Autodesk Inventor part; units mm, degrees
ref_plane "工作平面1" through (0, 10, 0) normal (0, 1, 0) x (-1, 0, 0)
ref_plane "YZ Plane" through (0, 0, 0) normal (1, 0, 0) x (0, 1, 0)
ref_plane "XY Plane" through (0, 0, 0) normal (0, 0, 1) x (1, 0, 0)
sketch "草图1" plane through (0, 0, 0) normal (0, 1, 0) x (-1, 0, 0)
  line L0 (10, -52.5) -> (-10, -52.5)
  line L1 (-10, -52.5) -> (-10, 52.5)
  line L2 (-10, 52.5) -> (10, 52.5)
  line L3 (10, 52.5) -> (10, -52.5)
  line L4 (10, -52.5) -> (-10, 52.5) construction
  line L5 (-10, -52.5) -> (10, 52.5) construction
  point P0 (0, 0)
  dimension "d0" = 20
  dimension "d1" = 105
extrude "拉伸1" add sketch "草图1" along normal blind 25
sketch "草图3" plane through (0, 25, 0) normal (0, 1, 0) x (1, 0, 0)
  line L0 (10, -52.5) -> (10, 52.5)
  line L1 (10, 52.5) -> (-10, 52.5)
  line L2 (-10, 52.5) -> (-10, -52.5)
  line L3 (-10, 52.5) -> (-10, -52.5)
  line L4 (-10, -52.5) -> (10, -52.5)
  line L5 (10, -52.5) -> (10, 52.5)
  line L6 (-10, 52.5) -> (-10, -28.5)
  line L7 (-10, -24.5) -> (10, -24.5)
  line L8 (10, -52.5) -> (10, 52.5)
  line L9 (10, 52.5) -> (-10, 52.5)
  line L10 (-10, -52.5) -> (10, -52.5)
  point P0 (0, 0)
  point P1 (10, -28.5)
  point P2 (10, -48.5)
  dimension "d12" = 28
extrude "拉伸3" cut sketch "草图3" against normal blind 5 contours L7 L2 L1 L0
sketch "草图4" plane through (0, 20, 0) normal (0, 1, 0) x (1, 0, 0)
  point P0 (0, 0)
sketch "草图6" plane through (0, 0, 0) normal (1, 0, 0) x (0, 1, 0)
  line L0 (0, -52.5) -> (20, -52.5)
  line L1 (0, -52.5) -> (0, 52.5)
  circle A0 centre (10, 4.5) radius 6
  point P0 (0, 0)
  point P1 (15, -52.5)
  dimension "d18" = 57
  dimension "d19" = 10
  dimension "d20" = 12
extrude "拉伸5" cut sketch "草图6" along normal mid plane 19
ref_plane "工作平面1" through (0, 10, 0) normal (0, 1, 0) x (-1, 0, 0)
sketch "草图8" plane through (0, 10, 0) normal (0, 1, 0) x (-1, 0, 0)
  line L0 (10, 52.5) -> (-10, 52.5)
  line L1 (10, -52.5) -> (10, 52.5)
  line L2 (-10, -52.5) -> (10, -52.5)
  line L3 (-10, 52.5) -> (-10, -52.5)
  line L4 (9.5, -1.5) -> (9.5, 10.5)
  line L5 (-9.5, 10.5) -> (-9.5, -1.5)
  line L6 (9.5, -1.5) -> (9.5, 10.5)
  line L7 (9.5, 4.5) -> (10, 4.5)
  line L8 (10, -52.5) -> (10, 52.5)
  line L9 (9.5, -1.5) -> (10, -2)
  line L10 (10, -2) -> (10, 4.5)
  line L11 (9.5, 4.5) -> (9.5, -1.5)
  line L12 (10, 4.5) -> (-10, 4.5)
  line L13 (-10, 52.5) -> (-10, -52.5)
  point P0 (0, 0)
  dimension "d24" = 135
revolve "旋转1" cut sketch "草图8" angle 360 about axis through (-10, 10, 4.5) along (1, 0, 0) contours L1 L9 L4 L7
mirror "镜像1" about plane through (0, 0, 0) normal (1, 0, 0) of "旋转1"
sketch "草图9" plane through (0, 0, 0) normal (1, 0, 0) x (0, 1, 0)
  line L0 (0, -52.5) -> (20, -52.5)
  line L1 (25, 24.5) -> (25, 52.5)
  line L2 (14.5, 38.5) -> (31.5646, 38.5)
  line L3 (14.5, 38.5) -> (14.5, 37)
  line L4 (14.5, 37) -> (16.5, 37)
  line L5 (16.5, 37) -> (25, 28.5)
  line L6 (25, 28.5) -> (25, 38.5)
  line L7 (25, 52.5) -> (25, 24.5)
  line L8 (14.5, 40) -> (16.5, 40)
  line L9 (16.5, 40) -> (25, 48.5)
  line L10 (14.5, 40) -> (14.5, 38.5)
  point P0 (0, 0)
  point P1 (15, -52.5)
  dimension "d26" = 91
  dimension "d27" = 10.5
  dimension "d28" = 1.5
  dimension "d29" = 2
  dimension "d30" = 45
extrude "拉伸6" cut sketch "草图9" along normal through all both and the other way through all
sketch "草图10" plane through (0, 20, 0) normal (0, 1, 0) x (1, 0, 0)
  line L0 (-10, 52.5) -> (-10, -52.5)
  line L1 (-10, 17.5) -> (10, 17.5)
  line L2 (10, -52.5) -> (10, 52.5)
  line L3 (-10, 52.5) -> (10, 52.5)
  circle A0 centre (0, 17.5) radius 7
  line L4 (-7, 17.5) -> (-7, 52.5)
  line L5 (10, 52.5) -> (-10, 52.5)
  line L6 (7, 17.5) -> (6.4266, 52.5)
  point P0 (0, 0)
  point P1 (6.9962, 17.7293)
  dimension "d33" = 35
  dimension "d34" = 14
extrude "拉伸7" cut sketch "草图10" against normal blind 5 contours L3 L6 L1 L4 | L1 A0
properties part number "5-压铁" material "不锈钢"
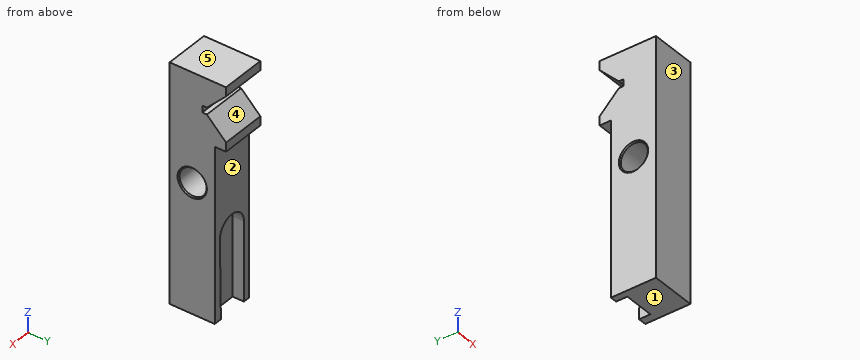
Part model, mm, in its own coordinate system. Face numbers are marked on the shaded views. A direction names the side the tool comes from. Coordinates: 2 decimals unless noted, no trailing zeros. Loops run counter-clockwise (first coordinate to the right, second up) from the corner with the lowest first, then second, coordinate; pieces in that order, holes last. Notation, with made-up numbers: (18.5, -13) - (49.5, -13) arc R13 cw to (49.5, 0) - close; hole circle Ø8 at (80.5, 57.25). An arc over 180 degrees is marked (long way). Write item = value, one per line. Start each with the question number.
Item 1: Cut at A-A, the plane y = 10. Give the cut face in (x, z), and give its area (3 significant figures).
Item 2: Cut at D-D, the plane z = 38.5. Give the cut face in (x, y), and give its area (3 significant figures).
Item 3: 3-axis set-ups, long thin cutter, end or side, ignore diameter. For the marked faces 1 and 2: which of +Z, -Z, +X, -X, +Y, -Y reach the whole face in a straight line?
Item 4: Cut at B-B, the plane z = 4.5. Give the cut face in (x, y).
Item 5: Wall check: L1, parallel to Z at x = -5.5, y = 10; L2, parallel to Y at x = -4.75, z = 4.5; L3, parallel to Y at x = -8.25, z = 2. Give the ranges that are in metal, low to high. Write a range as from..to.
Item 6: Mould opens along Z. For the marked faces 3, 4 and 5 say: released by +Z, released by -Z, zero draft, split by the parting line, or undercut.
Item 7: Cut at C-C, the plane x = 0. Give the cut face in (y, z), and give its area (3 significant figures).
Item 8: Flat gauge pins, fed straight in: pin 1 Ø7 at (x, z) = (-2, -28.5) entering from +Y; pin 2 Ø0.9 at (x, z) = (-4.5, 39) entering from +Y; pin 3 Ø2.5 at (x, y) = (1, 22) entering from -Z. Where does each tip first touch, or does it go through?
The answers:
q1.outline = (-10, -52.5) - (10, -52.5) - (10, -2) - (9.5, -1.5) - (-9.5, -1.5) - (-10, -2) - close; (-10, 11) - (-9.5, 10.5) - (9.5, 10.5) - (10, 11) - (10, 52.5) - (-10, 52.5) - close
q1.area = 1,860 mm2
q2.outline = (-10, 0) - (10, 0) - (10, 14.5) - (-10, 14.5) - close
q2.area = 290 mm2
q3.face_1 = -Z, +X, -X, +Y, -Y
q3.face_2 = -Z, +X, -X, +Y
q4.outline = (-10, 0) - (10, 0) - (10, 3.5) - (9.5, 4) - (-9.5, 4) - (-10, 3.5) - close; (-10, 16.5) - (-9.5, 16) - (9.5, 16) - (10, 16.5) - (10, 20) - (-10, 20) - close
q5.L1 = -52.5..-1.5, 10.5..52.5
q5.L2 = 0..4, 16..20
q5.L3 = 0..4.55, 15.45..20
q6.face_3 = zero draft
q6.face_4 = undercut
q6.face_5 = released by +Z
q7.outline = (0, -52.5) - (15, -52.5) - (15, -10.5) - (20, -10.5) - (20, 24.5) - (25, 24.5) - (25, 28.5) - (16.5, 37) - (14.5, 37) - (14.5, 40) - (16.5, 40) - (25, 48.5) - (25, 52.5) - (0, 52.5) - close; hole circle Ø12 at (10, 4.5)
q7.area = 1,810 mm2
q8.pin_1 = 15
q8.pin_2 = 14.5
q8.pin_3 = 24.5
